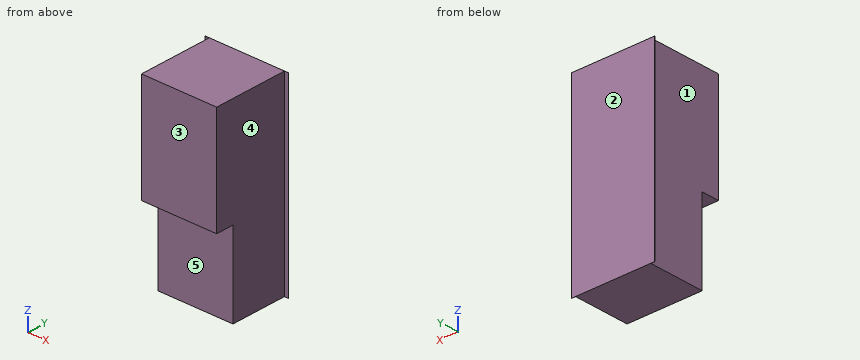
from build123d import *

# Parameters (mm, degrees)
F0_W     = 465
F0_H     = 1065
F1_DEPTH = 1
F2_W     = 420
F2_H     = 1065
F3_DEPTH = 315
F4_W     = 420
F4_H     = 598
F5_DEPTH = 100


with BuildPart() as f1:
    # F0 (on Front) → F1 (new body)
    with BuildSketch(Plane.XZ):
        Rectangle(F0_W, F0_H)
    extrude(amount=F1_DEPTH)

    # F2 (on face) → F3 (join)
    with BuildSketch(Plane.XZ.offset(1)):
        Rectangle(F2_W, F2_H)
    extrude(amount=F3_DEPTH)

    # F4 (on face) → F5 (join)
    with BuildSketch(Plane.XZ.offset(316)):
        with Locations((0, 233.5)):
            Rectangle(F4_W, F4_H)
    extrude(amount=F5_DEPTH)


solid = f1.part
Geometry: final body of the model. Coordinates: model frame, mm. Face numbers are marked on the shaded views. A direction names the side the tool comes from. Give positions to 0.01 mm unless a question says otherwise; leave off trailing zeros. Loops run counter-clockwise (first coordinate to the right, second up) from the corner with the lowest first, then second, coordinate; pieces in that order, holes last. Notation, with made-up numbers: (34, 60) -> (84, 60) arc R22 cw to (84, 85) -> close; hole circle Ø3 at (57, 62.5). An arc over 180 degrees is marked (long way). Put each result on its own line as item: value.
1. Cut plane B-B (x = 46.5). Return the cut outline in (y, z), plus the area to 3 significant figures.
Taken from the geometry:
outline: (-416, -65.5) -> (-316, -65.5) -> (-316, -532.5) -> (0, -532.5) -> (0, 532.5) -> (-416, 532.5) -> close
area: 396,000 mm2
2. Ray query, line 1 along X through (y, z) = (-178, 132); line 2 along Y through (x, z) = (-179, -456); line 3 along Z through (x, y) = (60, -398). Return the intervals inside material, ascending. Write a range as [from, to].
Taken from the geometry:
line 1: x = [-210, 210]
line 2: y = [-316, 0]
line 3: z = [-65.5, 532.5]
3. Set-up query: the marked faces 1, 2, 3, 4 and 5. Return all of +Z, -Z, +X, -X, +Y, -Y with unobstructed straight access to the full face (end or side cutting, diameter ignored); none if empty.
Taken from the geometry:
face 1: +Z, -Z, -X, -Y
face 2: +Z, -Z, +X, -X, +Y
face 3: +Z, -Z, +X, -X, -Y
face 4: +Z, -Z, +X, -Y
face 5: -Z, +X, -X, -Y
4. Pin query (flat end, axial travel): P1, Ø11, axis at x = 219, z = -218, coming from the -Y side; P2, Ø12, axis at y = -207, z = 58, coming from the -X side; P3, Ø1, axis at y = -111.5, z = -124.5, coming from the +X side. Return the tip coordinate at first contact, or that it passes through.
Taken from the geometry:
P1: stops at y = -1
P2: stops at x = -210
P3: stops at x = 210
5. Cut plane A-A (z = -433). Return the cut outline in (x, y).
Taken from the geometry:
outline: (-232.5, -1) -> (-210, -1) -> (-210, -316) -> (210, -316) -> (210, -1) -> (232.5, -1) -> (232.5, 0) -> (-232.5, 0) -> close
6. Cut plane C-C (z = 102). Return the cut outline in (x, y), plus the area to 3 significant figures.
Taken from the geometry:
outline: (-232.5, -1) -> (-210, -1) -> (-210, -416) -> (210, -416) -> (210, -1) -> (232.5, -1) -> (232.5, 0) -> (-232.5, 0) -> close
area: 175,000 mm2
7. Cut plane D-D (y = -284). Return the cut outline in (x, z), plus the area to 3 significant figures.
Taken from the geometry:
outline: (-210, -532.5) -> (210, -532.5) -> (210, 532.5) -> (-210, 532.5) -> close
area: 447,000 mm2
